Part print with two shaded views. Sizes in mm from the minimum x, y, z corner. Coordinates: 2 decimals unless noted, no trailing zeros. Loops run counter-clockwise (first coordinate to the right, second up) from the corner with the lowest first, then second, coordinate; pieces in that order, holes last. Notation, with made-up numbers: (66.5, -30.5) -> (115.5, -30.5) arc R15 cw to (115.5, -22.5) -> close; hole circle Ø2 at (78, 88). An arc over 180 degrees is marked (long way). Use one line per item in the form item = value.
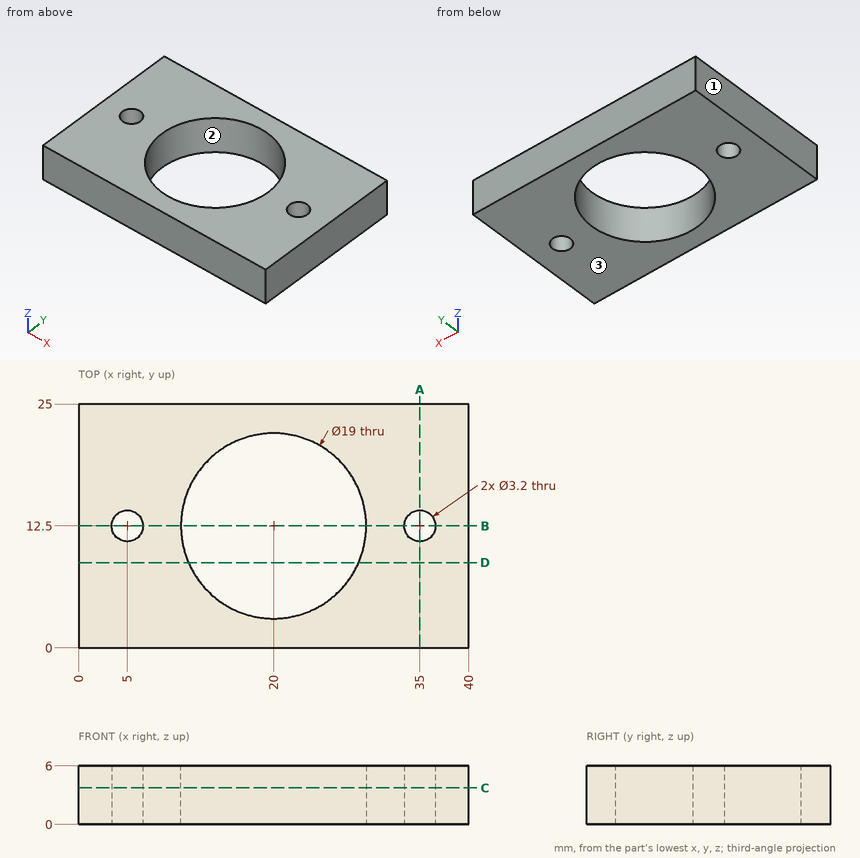
Q1. Band-saw the part on B-B, the plane y = 12.5. Write the cut outline in (x, z), and give its area (3 significant figures).
Result:
outline = (0, 0) -> (3.4, 0) -> (3.4, 6) -> (0, 6) -> close; (6.6, 0) -> (10.5, 0) -> (10.5, 6) -> (6.6, 6) -> close; (29.5, 0) -> (33.4, 0) -> (33.4, 6) -> (29.5, 6) -> close; (36.6, 0) -> (40, 0) -> (40, 6) -> (36.6, 6) -> close
area = 87.6 mm2
Q2. Band-saw the part on A-A, the plane x = 35. Write the cut outline in (y, z).
Result:
outline = (0, 0) -> (10.9, 0) -> (10.9, 6) -> (0, 6) -> close; (14.1, 0) -> (25, 0) -> (25, 6) -> (14.1, 6) -> close
Q3. Band-saw the part on C-C, the plane z = 3.75. Write the cut outline in (x, y).
Result:
outline = (0, 0) -> (40, 0) -> (40, 25) -> (0, 25) -> close; hole circle Ø3.2 at (5, 12.5); hole circle Ø19 at (20, 12.5); hole circle Ø3.2 at (35, 12.5)
Q4. Mould opens along X. For the marked faces 1, 2 and 3 say: released by +X, released by -X, zero draft, split by the parting line, or undercut.
Result:
face_1 = released by -X
face_2 = undercut
face_3 = zero draft
Q5. Wall check: line 1 along Y through (x, z) = (5, 2.7); line 2 along X through (y, z) = (12, 5.1); line 3 along X through (y, z) = (11.25, 2.4). Give the ranges that are in metal, low to high.
Result:
line_1 = 0 to 10.9, 14.1 to 25
line_2 = 0 to 3.48, 6.52 to 10.51, 29.49 to 33.48, 36.52 to 40
line_3 = 0 to 4, 6 to 10.58, 29.42 to 34, 36 to 40
Q6. Pin check, flat tip, straight feed: pin 1 Ø3 at (x, y) = (35, 12.5) entering from +Z. Stop position of the tip, or through.
Result:
pin_1 = through
Q7. Band-saw the part on D-D, the plane y = 8.75. Write the cut outline in (x, z), and give its area (3 significant figures).
Result:
outline = (0, 0) -> (11.27, 0) -> (11.27, 6) -> (0, 6) -> close; (28.73, 0) -> (40, 0) -> (40, 6) -> (28.73, 6) -> close
area = 135 mm2
